Build history of the part. All positions in model axes, mm. Face numbers are marked on the shaded views. A direction names the side the tool comes from. Round coordinates to 2 decimals unless told otherwise and drop trailing zeros. Write each loop counter-clockwise with the first axis right and the second up, starting at its lowest first coordinate (ties: lowest second). Pieces come first, ordered by that corner, then holes. Notation, with made-up numbers: (-29.75, 69) -> (-21.75, 69) arc R35 ccw to (-21.75, 102) -> close; hole circle Ø10 at (69, 8.25). An arc over 180 degrees is marked (long way). Answer in a Markdown table with one row per item.
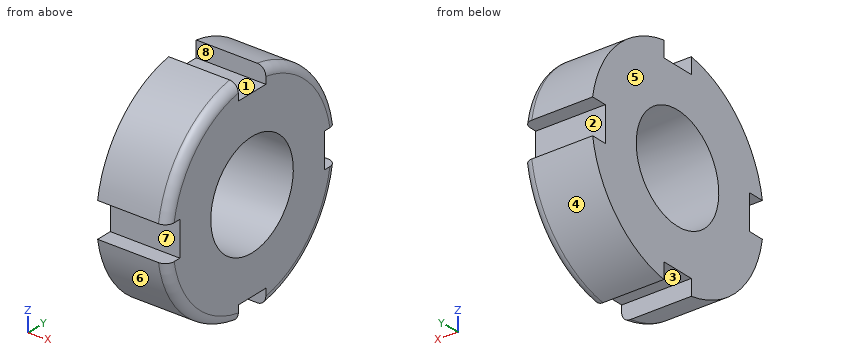
```python
from build123d import *

# Parameters (mm, degrees)
SKETCH1_R           = 12.5
BOSS_EXTRUDE1_DEPTH = 8
SKETCH2_R           = 6
CUT_EXTRUDE1_DEPTH  = 9
FILLET1_R           = 1
SKETCH3_W           = 4
SKETCH3_H           = 4
CUT_EXTRUDE2_DEPTH  = 9
CIRPATTERN1_COUNT   = 4


with BuildPart() as part:
    # Sketch1 → Boss-Extrude1 (new body)
    with BuildSketch(Plane(origin=(0, 0, 0), x_dir=(0, 0, -1), z_dir=(1, 0, 0))):
        Circle(SKETCH1_R)
    extrude(amount=BOSS_EXTRUDE1_DEPTH)

    # Sketch2 → Cut-Extrude1 (cut, through all)
    with BuildSketch(Plane(origin=(8, 0, 0), x_dir=(0, 0, -1), z_dir=(1, 0, 0))):
        Circle(SKETCH2_R)
    extrude(amount=-CUT_EXTRUDE1_DEPTH, mode=Mode.SUBTRACT)

    # Fillet1
    fillet1_edges = [part.edges().sort_by_distance(p)[0] for p in [
        (8, 0, 12.5),
    ]]
    fillet(fillet1_edges, radius=FILLET1_R)

    # Sketch3 → Cut-Extrude2 (cut, through all)
    with BuildSketch(Plane(origin=(8, 0, 0), x_dir=(0, 0, -1), z_dir=(1, 0, 0))):
        with Locations((0, 12.5)):
            Rectangle(SKETCH3_W, SKETCH3_H)
    cut_extrude2 = extrude(amount=-CUT_EXTRUDE2_DEPTH, mode=Mode.SUBTRACT)

    # CirPattern1: Cut-Extrude2 ×4 about axis
    cirpattern1_axis = Axis((0, 0, 0), (1, 0, 0))
    for i in range(1, CIRPATTERN1_COUNT):
        add(cut_extrude2.rotate(cirpattern1_axis, i * 360 / CIRPATTERN1_COUNT), mode=Mode.SUBTRACT)


solid = part.part
```
Q1. Which spindle directions (+Z, -Z, +X, -X, +Y, -Y) get a long thin tool onto all of the face, cutting with end or side? Do the marked faces 1, 2, 3, 4 and 5. Say none if no direction does.
A:
| item | result |
|---|---|
| face 1 | +Z, +X, -X |
| face 2 | +X, -X, +Y |
| face 3 | -Z, +X, -X |
| face 4 | -Z, +X, -X, +Y |
| face 5 | +Z, -Z, -X, +Y, -Y |
Q2. Drop flat-ended pins along their axis: P1, Ø3, axis at y = -7, z = 5, coming from the -X side; P2, Ø2, axis at x = 3.5, z = -11, coming from the +Y side; P3, Ø2, axis at x = 5, y = -12, coming from the +Z side; P4, Ø4.5, axis at x = 5, z = -0.5, coming from the -Y side. Give the stop position or say it passes through.
A:
| item | result |
|---|---|
| P1 | x = 0 |
| P2 | y = 7.5 |
| P3 | z = 5.94 |
| P4 | y = -12.34 |
Q3. Saw through at A-A on z = 0. Write the cut outline in (x, y).
A:
| item | result |
|---|---|
| outline | (0, -10.5) -> (8, -10.5) -> (8, -6) -> (0, -6) -> close; (0, 6) -> (8, 6) -> (8, 10.5) -> (0, 10.5) -> close |
Q4. Saw through at C-C on x = 6.5. Write the cut outline in (y, z).
A:
| item | result |
|---|---|
| outline | (-12.34, -2) arc R12.5 ccw to (-2, -12.34) -> (-2, -10.5) -> (2, -10.5) -> (2, -12.34) arc R12.5 ccw to (12.34, -2) -> (10.5, -2) -> (10.5, 2) -> (12.34, 2) arc R12.5 ccw to (2, 12.34) -> (2, 10.5) -> (-2, 10.5) -> (-2, 12.34) arc R12.5 ccw to (-12.34, 2) -> (-10.5, 2) -> (-10.5, -2) -> close; hole circle Ø12 at (0, 0) |
Q5. Two-plate mould, pull along Z, no slides. Class the marked faces 6, 7 and 8: released by +Z, released by -Z, zero draft, split by the parting line, or undercut.
A:
| item | result |
|---|---|
| face 6 | released by -Z |
| face 7 | undercut |
| face 8 | zero draft |
Q6. Wall check: line 1 (Y direction, x = 3.75, z = 0); line 2 (Y direction, x = 2.25, z = 1); line 3 (Z direction, x = 5, y = 3.5). Give the ranges that are in metal, low to high. Write a range as [from, to].
A:
| item | result |
|---|---|
| line 1 | [-10.5, -6], [6, 10.5] |
| line 2 | [-10.5, -5.92], [5.92, 10.5] |
| line 3 | [-12, -4.87], [4.87, 12] |
